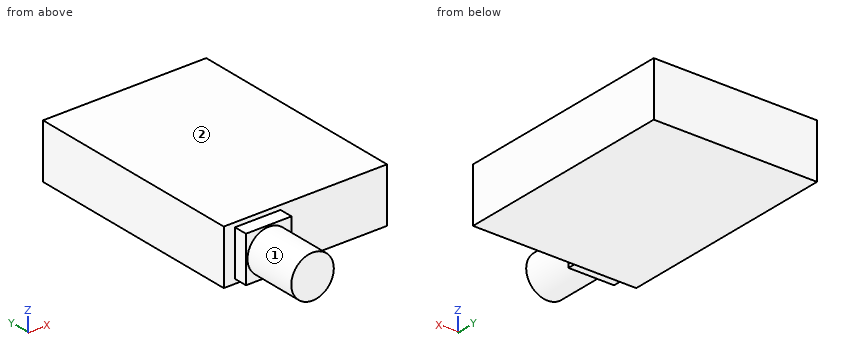
```python
from build123d import *

# Parameters (mm, degrees)
F0_W     = 24
F0_H     = 33
F1_DEPTH = 8
F2_W     = 6.7
F2_H     = 6.7
F3_DEPTH = 2
F4_R     = 3.125
F5_DEPTH = 8


with BuildPart() as f1:
    # F0 (on Top) → F1 (new body)
    with BuildSketch(Plane.XY):
        Rectangle(F0_W, F0_H)
    extrude(amount=F1_DEPTH)

    # F2 (on face) → F3 (join)
    with BuildSketch(Plane.XZ.offset(16.5)):
        with Locations((-7, 4)):
            Rectangle(F2_W, F2_H)
    extrude(amount=F3_DEPTH)

    # F4 (on face) → F5 (join)
    with BuildSketch(Plane.XZ.offset(18.5)):
        with Locations((-7, 4)):
            Circle(F4_R)
    extrude(amount=F5_DEPTH)


solid = f1.part
```
Verification items for the finished model (mm, model axes). Face numbers are marked on the shaded views. A direction names the side the tool comes from. Give positions to 0.01 mm unless a question says otherwise; leave off trailing zeros. Order: outer loops, then holes, each group sorted by start corner. A loop starts at its lowest first (then second) coordinate and runs counter-clockwise, first axis right, second up. Notation, with made-up numbers: M 37.25,-1.75 L 42.25,-1.75 A20 ccw 42.25,25.25 Z; hole C 38,34 d4. An arc over 180 degrees is marked long. Return JSON: item names as keys, results as strings. Group by question number.
1) Section check A-A on z = 4. Record the cut outline in (x, y) (3 decimals), and give its area (3 significant figures).
2) Scan lines: line 1 (Y direction, x = -3.5, z = 0.75); line 2 (Z direction, x = -7.5, y = -19.5); line 3 (X direction, y = -22.5, z = 5.75). Record each from-to range of solid material in increasing order.
3) Access from +Z, -Z, +X, -X, +Y, -Y to the whole of each face (thin tool, end or side, straight path). Record for the marked faces 1 and 2.
4) Section check B-B on x = -7. Record the cut outline in (y, z) (3 decimals), and give its area (3 significant figures).
5) Section check C-C on x = 9.25. Record the cut outline in (y, z).
6) Go/stop test with flat-tipped pins: pin 1 Ø1.6 at (x, y) = (-7, -17.5) entering from +Z; pin 2 Ø0.6 at (y, z) = (-18, 5.5) entering from -X; pin 3 Ø1 at (x, y) = (-6, -17.5) entering from -Z. Record where each tip stops, or that it passes through.
Answer block:
{
 "1": {"outline": "M -12,-16.5 L -10.35,-16.5 L -10.35,-18.5 L -10.125,-18.5 L -10.125,-26.5 L -3.875,-26.5 L -3.875,-18.5 L -3.65,-18.5 L -3.65,-16.5 L 12,-16.5 L 12,16.5 L -12,16.5 Z", "area": "855 mm^2"},
 "2": {"line 1": "y = -16.5 to 16.5", "line 2": "z = 0.92 to 7.08", "line 3": "x = -9.59 to -4.41"},
 "3": {"face 1": "-Y", "face 2": "+Z, +X, -X, +Y, -Y"},
 "4": {"outline": "M -26.5,0.875 L -18.5,0.875 L -18.5,0.65 L -16.5,0.65 L -16.5,0 L 16.5,0 L 16.5,8 L -16.5,8 L -16.5,7.35 L -18.5,7.35 L -18.5,7.125 L -26.5,7.125 Z", "area": "327 mm^2"},
 "5": {"outline": "M -16.5,0 L 16.5,0 L 16.5,8 L -16.5,8 Z"},
 "6": {"pin 1": "stops at z = 7.35", "pin 2": "stops at x = -10.35", "pin 3": "stops at z = 0.65"}
}
